Part print with two shaded views. Sizes in mm from the minimum x, y, z corner. Coordinates: 2 decimals unless noted, no trailing zeros. Order: outer loops, then holes, each group sorted by start corner. A loop starts at its lowest first (then second) coordinate and runs counter-clockwise, first axis right, second up.
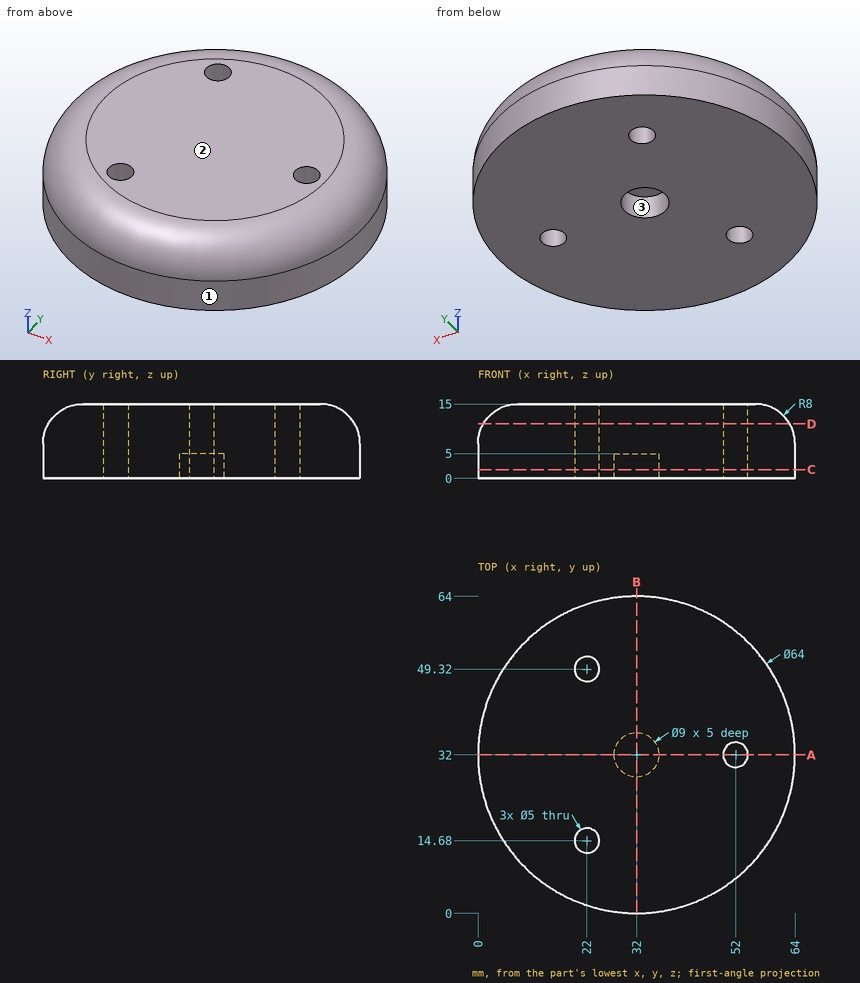
Q1. Cut at A-A on y = 32. Write the cut outline in (x, z).
Results list:
outline: (0, 0) - (27.5, 0) - (27.5, 5) - (36.5, 5) - (36.5, 0) - (49.5, 0) - (49.5, 15) - (8, 15) arc R8 ccw to (0, 7) - close; (54.5, 0) - (64, 0) - (64, 7) arc R8 ccw to (56, 15) - (54.5, 15) - close
Q2. Cut at C-C on z = 1.75. Write the cut outline in (x, y).
Results list:
outline: circle Ø64 at (32, 32); hole circle Ø5 at (22, 14.68); hole circle Ø5 at (22, 49.32); hole circle Ø9 at (32, 32); hole circle Ø5 at (52, 32)
Q3. Cut at D-D on z = 11. Write the cut outline in (x, y).
Results list:
outline: circle Ø61.86 at (32, 32); hole circle Ø5 at (22, 14.68); hole circle Ø5 at (22, 49.32); hole circle Ø5 at (52, 32)
Q4. Cut at B-B on x = 32. Write the cut outline in (y, z).
Results list:
outline: (0, 0) - (27.5, 0) - (27.5, 5) - (36.5, 5) - (36.5, 0) - (64, 0) - (64, 7) arc R8 ccw to (56, 15) - (8, 15) arc R8 ccw to (0, 7) - close
Q5. Wall check: line 1 along Y through (x, z) = (22, 10.5); line 2 along Y through (x, z) = (22, 7.25); line 3 along Y through (x, z) = (32, 3.85). Give the ranges that are in metal, low to high.
Results list:
line 1: y = 2.45 to 12.18, 17.18 to 46.82, 51.82 to 61.55
line 2: y = 1.61 to 12.18, 17.18 to 46.82, 51.82 to 62.39
line 3: y = 0 to 27.5, 36.5 to 64
Q6. Pin check, flat tips, straight feed: pin 1 Ø1.5 at (y, z) = (12, 7.5) entering from +X (1 decimal); pin 2 Ø3 at (x, y) = (22, 49.32) entering from -Z; pin 3 Ø6 at (y, z) = (55, 11.5) entering from +X; pin 4 Ø1 at (x, z) = (8, 4) entering from -Y. Stop position of each tip, or through.
Results list:
pin 1: stops at x = 57.5
pin 2: passes through
pin 3: stops at x = 55.89
pin 4: stops at y = 10.28
Q7. Mould opens along X. For the marked faces 1, 2 and 3 say: pulls with the +X half, pulls with the -X half, needs draft (parallel to the pull), parting line crosses it, or undercut.
Results list:
face 1: parting line crosses it
face 2: needs draft
face 3: undercut
